Build history of the part. All positions in model axes, mm. A direction names the side the tool comes from. Round coordinates to 2 decimals unless told otherwise and drop trailing zeros. Write each loop counter-clockwise with the first axis right and the second up, starting at its lowest first coordinate (ties: lowest second). Pieces come first, ordered by that corner, then holes. Notation, with made-up numbers: (79, 75.25) -> (130, 75.25) arc R25 ccw to (130, 109.25) -> close; hole circle Ø10 at (1, 14.25). An arc over 180 degrees is marked (long way). Return JSON: item names as keys, results as strings.
Autodesk Inventor part; units mm, degrees
ref_plane "Work Plane1" through (1.525, 0, 0) normal (0, 0, 1) x (1, 0, 0)
ref_plane "YZ Plane" through (0, 0, 0) normal (1, 0, 0) x (0, 1, 0)
ref_plane "XZ Plane" through (0, 0, 0) normal (0, 1, 0) x (-1, 0, 0)
sketch "Skizze1" plane through (0, 0, 0) normal (0, 0, 1) x (1, 0, 0)
  line L0 (0, 2.95) -> (0, 1.8106)
  line L1 (2.1, 2) -> (55, 2)
  line L2 (55, 2) -> (55, 0)
  line L3 (55, 0) -> (-0.4001, 0)
  line L4 (-11.4801, 0) -> (66.08, 0)
  line L5 (-0.4001, 0) -> (-0.4001, 2.95)
  line L6 (-0.4001, 2.95) -> (0, 2.95)
  line L7 (2.1, 2) -> (1.6705, 1.8106)
  line L8 (1.6705, 1.8106) -> (0, 1.8106)
  line L9 (0, -0.59) -> (0, 3.54)
  dimension "d0" = 55
  dimension "d1" = 52.9
  dimension "d2" = 4
  dimension "d9" = 0.4001
  dimension "d10" = 5.9
  dimension "d13" = 0.4295
  dimension "d14" = 3.6211
revolve "Körper" add sketch "Skizze1" angle 360 about axis through (55, 0, 0) along (-1, 0, 0)
sketch "Skizze2" plane through (-0.4001, 0, 0) normal (-1, 0, 0) x (0, 0, 1)
  line L0 (0, 4.0415) -> (3.5, 2.0207)
  line L1 (3.5, 2.0207) -> (3.5, -2.0207)
  line L2 (3.5, -2.0207) -> (0, -4.0415)
  line L3 (0, -4.0415) -> (-3.5, -2.0207)
  line L4 (-3.5, -2.0207) -> (-3.5, 2.0207)
  line L5 (-3.5, 2.0207) -> (0, 4.0415)
  point P0 (0, 0)
  point P1 (0, 0)
  dimension "d11" = 7
extrude "Kopf" add sketch "Skizze2" along normal blind 2.4
sketch "Skizze4" plane through (0, 0, 0) normal (0, 0, 1) x (1, 0, 0)
  line L0 (-2.8001, 3.5) -> (-2.8001, 4.0415)
  line L1 (-2.8001, 4.0415) -> (-2.4875, 4.0415)
  line L2 (-2.4875, 4.0415) -> (-2.8001, 3.5)
  line L3 (-3.2801, 0) -> (0.0799, 0)
  line L4 (-0.4001, 4.0415) -> (-2.8001, 4.0415)
  line L5 (-2.8001, 2.0207) -> (-2.8001, 4.0415)
  dimension "d5" = 30
  dimension "d19" = 7
revolve "Fase1" cut sketch "Skizze4" angle 360 about axis through (-10, 0, 0) along (1, 0, 0)
thread "Gewinde"
chamfer "Fase2" distance 0.4294 distance2 0.4295 1 edges at (55, -2, 0) measured on face at (55, -0.499, 0.4421)
ref_plane "Work Plane1" through (1.525, 0, 0) normal (0, 0, 1) x (1, 0, 0)
equation "\"d0\" = NLG"
equation "\"d1\" = GEL"
equation "\"d2\" = GD"
equation "\"d10\" = SD2"
equation "\"d14\" = BDM"
equation "\"d11\" = SW"
equation "\"d3\" = KOH - SD"
equation "\"d5\" = ANG1"
equation "\"d19\" = SW0"
equation "\"d15\" = GEL"
equation "\"d6\" = -0.5 * SPD + 0.5 * GD"
equation "\"NLG\" = 55"
equation "\"GD\" = NND"
equation "\"BDM\" = 3.62111"
equation "\"KOH\" = 2.8"
equation "\"GEL\" = 52.9"
equation "\"SW\" = 7"
equation "\"SW0\" = 7"
equation "\"SPD\" = NND - 1.2269 * PTC"
equation "\"SD2\" = 5.9"
equation "\"SD\" = 0.4"
equation "\"ANG1\" = 30deg"
equation "\"GAL\" = 0.61345 * PTC"
equation "\"GUL\" = 0.61345 * PTC"
equation "\"RR\" = 0.2"
equation "\"GD1\" = THREADDIA - 1.2269 * PTC"
equation "\"THREADDIA\" = 4"
equation "\"TOA\" = 30deg"
equation "\"PTC\" = 0.7"
equation "\"NND\" = 4"
equation "\"E0\" = 1.155 * SW"
properties part number "DIN 933 - M4  x 55" material "Stahl, weich"
Q1. Saw through at A-A on x = 21. List the corners of the cut face in (y, z), then the cut area to 3 significant figures.
Verdict:
{"outline": "circle Ø4 at (0, 0)", "area": "12.6 mm²"}
Q2. Two-plate mould, pull along X, no slides. Class faces 1 (the conical face through (-2.724, 1.823, 3.141)), 2 (the cylindrical face through (0.8, -0.2, -1.8)), 3 (the flat face through (-0.4, -3, -1)), 4 (the cylindrical face through (29, 0, -2)): +X half, -X half, draft (parallel to the pull), parting line (faces both ways), or undercut.
Verdict:
{"face 1": "-X half", "face 2": "undercut", "face 3": "+X half", "face 4": "draft"}
Q3. Wall check: L1, parallel to X at y = 2.5, z = -1.5; L2, parallel to Y at x = 45.5, z = -1.25; L3, parallel to Y at x = 16.5, z = 1. Give the ranges that are in metal, low to high.
Verdict:
{"L1": "x = -2.8 to 0", "L2": "y = -1.56 to 1.56", "L3": "y = -1.73 to 1.73"}
Q4. 3-axis set-ups, long thin cutter, end or side, ignore diameter. For faces 5 (the cylindrical face through (-0.197, -2.947, 0.13)), 6 (the conical face through (-2.724, -3.632, 0.009)): which of +Z, -Z, +X, -X, +Y, -Y reach the whole face in a straight line?
Verdict:
{"face 5": "+X", "face 6": "-X, -Y"}
Q5. Pin check, flat tips, straight feed: pin 1 Ø4 at (x, z) = (7, -1.5) entering from -Y; pin 2 Ø1 at (x, y) = (45.5, 0) entering from -Z; pin 3 Ø4 at (x, z) = (36, -2.5) entering from -Y. Stop position of each tip, or through.
Verdict:
{"pin 1": "stops at y = -2", "pin 2": "stops at z = -2", "pin 3": "stops at y = -1.94"}
